from build123d import *

# Parameters (mm, degrees)
SKETCH1_W                      = 74.549
SKETCH1_H                      = 74.549
SKETCH1_R                      = 24.511
BOSS_EXTRUDE1_DEPTH            = 1.5875
BOSS_EXTRUDE1_DEPTH_BACK       = 1.5875
SKETCH15_W                     = 74.549
SKETCH15_H                     = 74.549
SKETCH15_R                     = 28.6131
BOSS_EXTRUDE11_DEPTH           = 1.5875
CUT_EXTRUDE1_START             = -4.175
SKETCH2_R                      = 3.429
CUT_EXTRUDE1_DEPTH             = 6.7625
MIRROR2_START                  = -4.175
MIRROR2_COPY_1_SKETCH_R        = 3.429
MIRROR2_COPY_1_DEPTH           = 6.7625
SKETCH14_W                     = 49.149
SKETCH14_H                     = 8.290530285
CUT_EXTRUDE6_DEPTH             = 2.5875
CUT_EXTRUDE6_DEPTH_BACK        = 4.175
FILLET2_R                      = 3.175
CUT_EXTRUDE8_REACH             = 3.587
CUT_EXTRUDE8_DIRECTION_2_DEPTH = 0.635
SKETCH18_R                     = 28.6131
CUT_EXTRUDE9_DEPTH             = 0.635


with BuildPart() as part:
    # Sketch1 → Boss-Extrude1 (new body, two sides)
    with BuildSketch(Plane.XY) as boss_extrude1_sk:
        Rectangle(SKETCH1_W, SKETCH1_H)
        Circle(SKETCH1_R, mode=Mode.SUBTRACT)
    extrude(amount=BOSS_EXTRUDE1_DEPTH)
    extrude(boss_extrude1_sk.sketch, amount=-BOSS_EXTRUDE1_DEPTH_BACK)

    # Sketch15 → Boss-Extrude11 (add)
    with BuildSketch(Plane.XY.offset(1.5875)):
        Rectangle(SKETCH15_W, SKETCH15_H)
        Circle(SKETCH15_R, mode=Mode.SUBTRACT)
    extrude(amount=BOSS_EXTRUDE11_DEPTH)

    # Sketch2 → Cut-Extrude1 (cut)
    with BuildSketch(Plane.XY.offset(1.5875).offset(CUT_EXTRUDE1_START)):
        with Locations((-31.75, 31.75)):
            Circle(SKETCH2_R)
    cut_extrude1 = extrude(amount=CUT_EXTRUDE1_DEPTH, mode=Mode.SUBTRACT)

    # Mirror1: Cut-Extrude1 across plane
    add(cut_extrude1.mirror(Plane(origin=(0, 0, 0), x_dir=(0, 0, 1), z_dir=(1, 0, 0))), mode=Mode.SUBTRACT)

    # Mirror2: Cut-Extrude1 across plane
    add(cut_extrude1.mirror(Plane.ZX), mode=Mode.SUBTRACT)

    # Mirror2 copy 1 sketch → Mirror2 copy 1 (cut)
    with BuildSketch(Plane(origin=(0, 0, 1.5875), x_dir=(-1, 0, 0), z_dir=(0, 0, 1)).offset(MIRROR2_START)):
        with Locations((-31.75, 31.75)):
            Circle(MIRROR2_COPY_1_SKETCH_R)
    extrude(amount=MIRROR2_COPY_1_DEPTH, mode=Mode.SUBTRACT)

    # Sketch14 → Cut-Extrude6 (cut, two sides)
    with BuildSketch(Plane.XY.offset(1.5875)) as cut_extrude6_sk:
        with Locations((0, 35.069765143)):
            Rectangle(SKETCH14_W, SKETCH14_H)
    extrude(amount=CUT_EXTRUDE6_DEPTH, mode=Mode.SUBTRACT)
    extrude(cut_extrude6_sk.sketch, amount=-CUT_EXTRUDE6_DEPTH_BACK, mode=Mode.SUBTRACT)

    # Fillet2
    fillet2_edges = [part.edges().sort_by_distance(p)[0] for p in [
        (-24.5745, 30.9245, 0.79375),
        (24.5745, 30.9245, 0.79375),
    ]]
    fillet(fillet2_edges, radius=FILLET2_R)

    # Sketch17 → Cut-Extrude8 (cut, up to next)
    with BuildSketch(Plane.XY.offset(1.5875), mode=Mode.PRIVATE) as cut_extrude8_sk1:
        with BuildLine():
            Line((-1.5875, 24.754637718), (-1.5875, 33.858616052))
            ThreePointArc((-1.5875, 33.858616052), (0, 35.446116052), (1.5875, 33.858616052))
            Line((1.5875, 33.858616052), (1.5875, 24.754637718))
            ThreePointArc((1.5875, 24.754637718), (0, 23.167137718), (-1.5875, 24.754637718))
        make_face()
    cut_extrude8_tool1 = extrude(cut_extrude8_sk1.sketch, amount=CUT_EXTRUDE8_REACH, mode=Mode.PRIVATE) & part.part
    add(cut_extrude8_tool1.solids().sort_by_distance((0, 29.306627, 1.5875))[0], mode=Mode.SUBTRACT)

    # Sketch17 → Cut-Extrude8 direction 2 (cut)
    with BuildSketch(Plane.XY.offset(1.5875)):
        with BuildLine():
            Line((-1.5875, 24.754637718), (-1.5875, 33.858616052))
            ThreePointArc((-1.5875, 33.858616052), (0, 35.446116052), (1.5875, 33.858616052))
            Line((1.5875, 33.858616052), (1.5875, 24.754637718))
            ThreePointArc((1.5875, 24.754637718), (0, 23.167137718), (-1.5875, 24.754637718))
        make_face()
    extrude(amount=-CUT_EXTRUDE8_DIRECTION_2_DEPTH, mode=Mode.SUBTRACT)

    # Sketch18 → Cut-Extrude9 (cut)
    with BuildSketch(Plane.XY.offset(1.5875)):
        Circle(SKETCH18_R)
    extrude(amount=-CUT_EXTRUDE9_DEPTH, mode=Mode.SUBTRACT)


solid = part.part
The listing builds one solid part. Answer for the finished solid, in the listing's coordinates (mm). A direction names the side the tool comes from. Round coordinates to 2 decimals unless told otherwise and drop trailing zeros. Order: outer loops, then holes, each group sorted by start corner. A loop starts at its lowest first (then second) coordinate and runs counter-clockwise, first axis right, second up. Notation, with made-up numbers: M 54.5,72.5 L 65.5,72.5 A25 ccw 65.5,84.5 Z; hole C 0.25,-17 d3. An arc over 180 degrees is marked long. Answer in a Markdown table with one row per item. Add a question column.
1) The part is cut by section C-C on x = 0. Determine the outline of the cut face in (y, z) (1 decimal).
2) Which of the six approach directions +Z, -Z, +X, -X, +Y, -Y give full straight-line access (tool end or side, diameter ignored) to faces 1 (the face through (-1.588, 30, 2)), 2 (the face through (-24.574, 36, 1)), 3 (the face through (31, 37.274, 1)), 4 (the face through (-1.236, -28.586, 2.048)), 5 (the face through (28.48, -32.78, 0.76))?
3) Determine the mould class of faces 6 (the face through (-1, -37.274, 1)), 7 (the face through (-19.451, -14.915, -0.3)), 8 (the face through (13, 21, 0.952)), 9 (the face through (-37.274, -1, 1)) for opening direction Y: pulls with the +Y half, pulls with the -Y half, needs draft (parallel to the pull), parting line crosses it, or undercut.
4) Consider line 1 along Y through (x, z) = (31.75, 1.1); line 2 along Y through (x, z) = (-30.5, 0.1); line 3 along Y through (x, z) = (0, -0.5). Determine where each line is inside the solid, lowest interval first. Write a range as from..to.
5) Flat-ended cylindrical pins translate along their axes: pin 1 Ø1.5 at (x, z) = (23.5, 1) entering from +Y; pin 2 Ø2.5 at (x, z) = (5, 1) entering from +Y. Find the tip coordinate at first contact, or state that the pin passes through.
6) The part is cut by section B-B on y = 0. Determine the outline of the cut face in (x, z) (1 decimal), plus the area to 3 significant figures.
7) The part is cut by section A-A on x = 31.75. Determine the outline of the cut face in (y, z) (1 decimal), plus the area to 3 significant figures.
Findings below:
| question | item | result |
|---|---|---|
| 1 | outline | M -37.3,-1.6 L -24.5,-1.6 L -24.5,1 L -28.6,1 L -28.6,3.2 L -37.3,3.2 Z; M 24.5,-1.6 L 30.9,-1.6 L 30.9,1 L 24.5,1 Z |
| 2 | face 1 | +Z, +Y |
| 2 | face 2 | +Z, -Z, +Y |
| 2 | face 3 | +Z, -Z, +X, -X, +Y |
| 2 | face 4 | +Z |
| 2 | face 5 | +Z, -Z |
| 3 | face 6 | pulls with the -Y half |
| 3 | face 7 | undercut |
| 3 | face 8 | undercut |
| 3 | face 9 | needs draft |
| 4 | line 1 | y = -37.27..-35.18, -28.32..28.32, 35.18..37.27 |
| 4 | line 2 | y = -37.27..-34.94, -28.56..28.56, 34.94..37.27 |
| 4 | line 3 | y = -37.27..-24.51, 24.51..30.92 |
| 5 | pin 1 | stops at y = 32.7 |
| 5 | pin 2 | stops at y = 30.92 |
| 6 | outline | M -37.3,-1.6 L -24.5,-1.6 L -24.5,1 L -28.6,1 L -28.6,3.2 L -37.3,3.2 Z; M 24.5,-1.6 L 37.3,-1.6 L 37.3,3.2 L 28.6,3.2 L 28.6,1 L 24.5,1 Z |
| 6 | area | 103 mm² |
| 7 | outline | M -37.3,-1.6 L -35.2,-1.6 L -35.2,3.2 L -37.3,3.2 Z; M -28.3,-1.6 L 28.3,-1.6 L 28.3,3.2 L -28.3,3.2 Z; M 35.2,-1.6 L 37.3,-1.6 L 37.3,3.2 L 35.2,3.2 Z |
| 7 | area | 290 mm² |
